Source: CAD feature listing. Evaluate the final solid. Frame: model axes, mm. A direction names the side the tool comes from. Give positions to 0.01 mm unless a question says otherwise; leave off trailing zeros. Order: outer loops, then holes, each group sorted by start corner. A loop starts at its lowest first (then second) coordinate and runs counter-clockwise, first axis right, second up. Notation, with made-up numbers: M -6.5,87.5 L 37.5,87.5 A9 ccw 37.5,92.5 Z; hole C 13.25,32 d5. An arc over 180 degrees is marked long. Answer as a JSON object with one key per item and string values. Group by question number.
1. Section query D-D (x = -44.5). Output: boundary loops of the cut face in (y, z).
2. Section query B-B (x = -10). Output: boundary loops of the cut face in (y, z), plus the area to 3 significant figures.
3. Pin query (flat end, axial travel): P1, Ø2, axis at x = 3, z = 70.5, coming from the +Y side; P2, Ø1.5, axis at y = 45, z = 98, coming from the +X side; P3, Ø5, axis at x = -19, z = 73, coming from the -Y side; P4, Ø6, axis at x = -12.5, y = 41.5, coming from the -Z side. Return the tip coordinate at first contact, or that it passes through.
4. Material intervals for L1, parallel to Z at x = -33, y = 45; L2, parallel to Z at x = -7.5, y = 42; L3, parallel to X at y = 38, z = 55.5, sorted ascending. Write a range as [from, to].
5. Section query C-C (y = 37.5). Output: boundary loops of the cut face in (x, z).
6. Set-up query: faces 1 (the flat face through (-33, 37, 2)), 2 (the flat face through (-20.999, 54.5, 21.2)), 3 (the flat face through (-1, 40, 0)). Return all of +Z, -Z, +X, -X, +Y, -Y with unobstructed straight access to the full face (end or side cutting, diameter ignored); none if empty.
7. Pull-direction query (Z, two-part tool) for faces 4 (the flat face through (-1, 40, 120)), 5 (the flat face through (-51, 27, 46)), 6 (the flat face through (-1, 39, 118)); classes: +Z half, -Z half, draft (parallel to the pull), parting line (faces both ways), or undercut.
8. Section query A-A (z = 12). Output: boundary loops of the cut face in (x, y), plus the area to 3 significant figures.
from build123d import *

# Parameters (mm, degrees)
PAD_DEPTH    = 120
PAD001_DEPTH = 2
PAD002_DEPTH = 2
POCKET_DEPTH = 59.001


with BuildPart() as part:
    # Sketch → Pad (new body)
    with BuildSketch(Plane.XY):
        with BuildLine():
            ThreePointArc((52.459508, 27), (0, 59), (-52.459508, 27))
            Line((-52.459508, 27), (-50.199602, 27))
            ThreePointArc((50.199602, 27), (0, 57), (-50.199602, 27))
            Line((50.199602, 27), (52.459508, 27))
        make_face()
    extrude(amount=PAD_DEPTH)

    # Sketch001 → Pad001 (join)
    with BuildSketch(Plane.XY):
        with BuildLine():
            ThreePointArc((50.199602, 27), (0, 57), (-50.199602, 27))
            Line((-50.199602, 27), (50.199602, 27))
        make_face()
    extrude(amount=PAD001_DEPTH)

    # Sketch002 → Pad002 (join)
    with BuildSketch(Plane.XY.offset(118)):
        with BuildLine():
            ThreePointArc((50.199602, 27), (0, 57), (-50.199602, 27))
            Line((-50.199602, 27), (50.199602, 27))
        make_face()
    extrude(amount=PAD002_DEPTH)

    # Sketch003 → Pocket (cut, through all)
    with BuildSketch(Plane.XZ):
        with BuildLine():
            Line((-20.999165, 1.820858), (20.999236, 1.820858))
            Line((20.999236, 1.820858), (20.999236, 40.820858))
            ThreePointArc((20.999236, 40.820858), (-0.004079, 62), (-20.999165, 40.8127))
            Line((-20.999165, 1.820858), (-20.999165, 40.8127))
        make_face()
    extrude(amount=-POCKET_DEPTH, mode=Mode.SUBTRACT)


solid = part.part
Answer sheet:
{
 "1": {"outline": "M 27,0 L 38.74,0 L 38.74,120 L 27,120 L 27,118 L 35.62,118 L 35.62,2 L 27,2 Z"},
 "2": {"outline": "M 27,0 L 58.15,0 L 58.15,1.82 L 27,1.82 Z; M 27,118 L 56.12,118 L 56.12,59.47 L 58.15,59.47 L 58.15,120 L 27,120 Z", "area": "238 mm^2"},
 "3": {"P1": "y = 58.97", "P2": "x = 39.02", "P3": "y = 52.79", "P4": "z = 0"},
 "4": {"L1": "[0, 2], [118, 120]", "L2": "[0, 1.82], [118, 120]", "L3": "[-45.13, -42.49], [42.49, 45.13]"},
 "5": {"outline": "M -45.55,0 L 45.55,0 L 45.55,120 L -45.55,120 Z; hole M -42.93,2 L -21,2 L -21,1.82 L 21,1.82 L 21,2 L 42.93,2 L 42.93,118 L -42.93,118 Z"},
 "6": {"face 1": "-Y", "face 2": "+Y, -Y", "face 3": "-Z, +X, -X, +Y, -Y"},
 "7": {"face 4": "+Z half", "face 5": "draft", "face 6": "undercut"},
 "8": {"outline": "M -52.46,27 L -50.2,27 A57 cw -21,52.99 L -21,55.14 A59 ccw Z; M 21,52.99 A57 cw 50.2,27 L 52.46,27 A59 ccw 21,55.14 Z", "area": "166 mm^2"}
}
